Source: three-view drawing plus pictorial views. Frame: mm from the lowest corner of the part. Give positions to 0.01 mm unless a question says otherwise; leave off trailing zeros. Order: outer loops, then holes, each group sorted by start corner. A loop starts at its lowest first (then second) coordinate and runs counter-clockwise, first axis right, second up. Notation, with made-up numbers: (-23, 89.25) -> (11, 89.25) arc R24 cw to (11, 110.25) -> close; hole circle Ø1 at (-10, -13). An arc over 180 degrees is marked (long way). One line per question, with ' | ' between items.
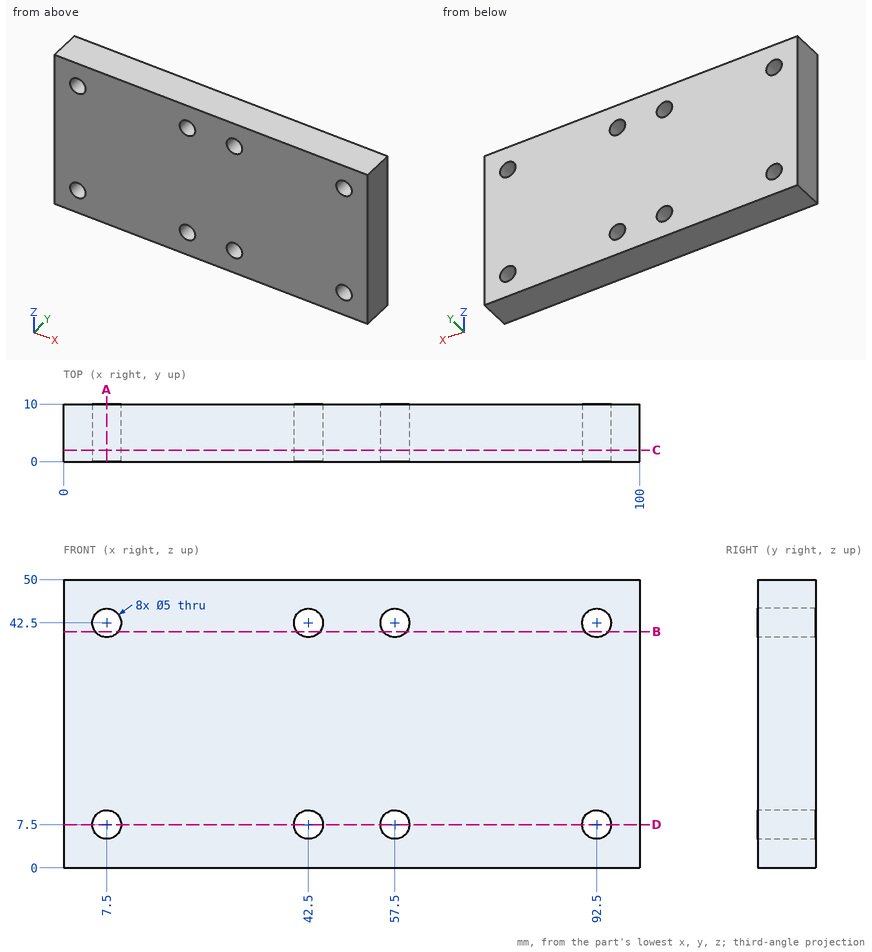
1) Section D-D on z = 7.5. Return loops of the section in (x, y).
Check result:
outline: (0, 0) -> (5, 0) -> (5, 10) -> (0, 10) -> close; (10, 0) -> (40, 0) -> (40, 10) -> (10, 10) -> close; (45, 0) -> (55, 0) -> (55, 10) -> (45, 10) -> close; (60, 0) -> (90, 0) -> (90, 10) -> (60, 10) -> close; (95, 0) -> (100, 0) -> (100, 10) -> (95, 10) -> close
2) Section A-A on x = 7.5. Return loops of the section in (y, z), plus the area to 3 significant figures.
Check result:
outline: (0, 0) -> (10, 0) -> (10, 5) -> (0, 5) -> close; (0, 10) -> (10, 10) -> (10, 40) -> (0, 40) -> close; (0, 45) -> (10, 45) -> (10, 50) -> (0, 50) -> close | area: 400 mm^2
3) Section C-C on y = 2. Count the separate pieces of the cut face and the enclosed holes in it, plus the area to 3 significant figures.
Check result:
separate pieces: 1 | enclosed holes: 8 | area: 4,840 mm^2
4) Section B-B on z = 41. Return loops of the section in (x, y), plus the area to 3 significant figures.
Check result:
outline: (0, 0) -> (5.5, 0) -> (5.5, 10) -> (0, 10) -> close; (9.5, 0) -> (40.5, 0) -> (40.5, 10) -> (9.5, 10) -> close; (44.5, 0) -> (55.5, 0) -> (55.5, 10) -> (44.5, 10) -> close; (59.5, 0) -> (90.5, 0) -> (90.5, 10) -> (59.5, 10) -> close; (94.5, 0) -> (100, 0) -> (100, 10) -> (94.5, 10) -> close | area: 840 mm^2
5) Contact query for a flat-ended pin moving along its axis: pin 1 Ø8 at (x, z) = (57.5, 42.5) entering from +Y. Output: stop coordinate, or through.
Check result:
pin 1: stops at y = 10
6) Material intervals for probe 1 along Z at (x, y) = (57.5, 6.75); probe 2 along X at (y, z) = (7, 42.5); probe 3 along X at (y, z) = (6.25, 42), sorted ascending. Write a range as from..to.
Check result:
probe 1: z = 0..5, 10..40, 45..50 | probe 2: x = 0..5, 10..40, 45..55, 60..90, 95..100 | probe 3: x = 0..5.05, 9.95..40.05, 44.95..55.05, 59.95..90.05, 94.95..100
